Can you work these out from the model? Positions are in its coordinate system, mm. Face numbers are marked on the shaded views. A direction names the side the tool comes from. Coordinates: 2 decimals unless noted, no trailing zeros. Write each loop counter-clockwise with the first axis right and the second up, starting at its lowest first coordinate (ties: lowest second). Pieces come first, ordered by that corner, then holes.
```python
from build123d import *

# Parameters (mm, degrees)
F1_DEPTH = 30
F2_W     = 3
F2_H     = 8
F3_DEPTH = 8
F4_R     = 3


with BuildPart() as f1:
    # F0 (on Top) → F1 (new body)
    with BuildSketch(Plane.XY):
        with BuildLine():
            ThreePointArc((11.5, 3.5), (9.156854, 9.156854), (3.5, 11.5))
            Line((3.5, 11.5), (-3.5, 11.5))
            ThreePointArc((-3.5, 11.5), (-9.156854, 9.156854), (-11.5, 3.5))
            Line((-11.5, 3.5), (-11.5, -3.5))
            ThreePointArc((-11.5, -3.5), (-9.156854, -9.156854), (-3.5, -11.5))
            Line((-3.5, -11.5), (3.5, -11.5))
            ThreePointArc((3.5, -11.5), (9.156854, -9.156854), (11.5, -3.5))
            Line((11.5, -3.5), (11.5, 3.5))
        make_face()
    extrude(amount=F1_DEPTH)

    # F2 (on Top) → F3 (join)
    with BuildSketch(Plane.XY):
        Rectangle(F2_W, F2_H)
    extrude(amount=-F3_DEPTH)

    # F4
    f4_edges = [f1.edges().sort_by_distance(p)[0] for p in [
        (-9.156854, -9.156854, 30),
        (9.156854, -9.156854, 0),
        (-1.5, 0, 0),
        (0, -4, 0),
        (1.5, 0, 0),
        (0, 4, 0),
        (0, 4, -8),
        (0, -4, -8),
    ]]
    fillet(f4_edges, radius=F4_R)


solid = f1.part
```
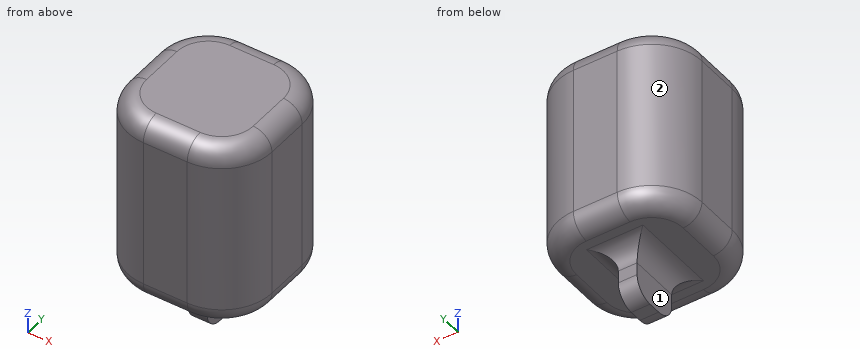
1. If we section it at C-C, the plane x = 2: List the corners of the cut face in (y, z) for me, plus the area to 3 significant figures.
2. If we section it at B-B, the plane z = 8: List the corners of the cut face in (x, y) for me, plus the area to 3 significant figures.
3. If we section it at A-A, the plane y = 0.25: List the corners of the cut face in (x, z) for me.
4. If we section it at D-D, the plane y = -3: List the corners of the cut face in (x, z) for me, plus the area to 3 significant figures.
5. I'm going to push flat-ended pins straight in: P1, Ø13.5, axis at x = 3, y = -0.5, coming from the -Z side; P2, Ø4, axis at y = -1, z = -5.5, coming from the +X side; P3, Ø5, axis at x = -3, z = -3.5, coming from the -Y side; P4, Ø0.6, axis at x = 0.5, z = -3.5, coming from the -Y side. Where does each tip first touch, or does it pass through?
6. If I drill on L1, parallel to Y at x = -0.75, z = -4; L2, parallel to Z at x = -6.75, y = -2; L3, parallel to X at y = -9.75, z = 12.5, over which ranges is the centre line in solid material (lowest first)?
7. Which directions (+Z, -Z, +X, -X, +Y, -Y) give clear straight access to the entire face, cutting with the end or side of a thin tool? Please do the marked faces 1 and 2.
Answers:
1. outline: (-11.5, 3) arc R3 ccw to (-8.5, 0) - (-7, 0) arc R3 cw to (-4.5, -1.34) - (4.5, -1.34) arc R3 cw to (7, 0) - (8.5, 0) arc R3 ccw to (11.5, 3) - (11.5, 27) arc R3 ccw to (8.5, 30) - (-8.5, 30) arc R3 ccw to (-11.5, 27) - close
1. area: 696 mm2
2. outline: (-11.5, -3.5) arc R8 ccw to (-3.5, -11.5) - (3.5, -11.5) arc R8 ccw to (11.5, -3.5) - (11.5, 3.5) arc R8 ccw to (3.5, 11.5) - (-3.5, 11.5) arc R8 ccw to (-11.5, 3.5) - close
2. area: 474 mm2
3. outline: (-11.5, 3) arc R3 ccw to (-8.5, 0) - (-4.5, 0) arc R3 cw to (-1.5, -3) - (-1.5, -8) - (1.5, -8) - (1.5, -3) arc R3 cw to (4.5, 0) - (8.5, 0) arc R3 ccw to (11.5, 3) - (11.5, 27) arc R3 ccw to (8.5, 30) - (-8.5, 30) arc R3 ccw to (-11.5, 27) - close
4. outline: (-11.5, 3) arc R3 ccw to (-8.5, 0) - (-4.5, 0) arc R3 cw to (-1.5, -3) - (-1.5, -7.24) - (1.5, -7.24) - (1.5, -3) arc R3 cw to (4.5, 0) - (8.5, 0) arc R3 ccw to (11.5, 3) - (11.5, 27) arc R3 ccw to (8.5, 30) - (-8.5, 30) arc R3 ccw to (-11.5, 27) - close
4. area: 708 mm2
5. P1: stops at z = -8
5. P2: stops at x = 1.5
5. P3: stops at y = -4.63
5. P4: stops at y = -4
6. L1: y = -4 to 4
6. L2: z = 0 to 30
6. L3: x = -8.49 to 8.49
7. face 1: -Z, -X, +Y, -Y
7. face 2: +Z, -Z, -X, +Y
